```python
from build123d import *

# Parameters (mm, degrees)
BOSS_EXTRUDE6_DEPTH = 4
CUT_EXTRUDE1_DEPTH  = 2


with BuildPart() as part:
    # Sketch2 → Boss-Extrude6 (new body)
    with BuildSketch(Plane.XY):
        with BuildLine():
            Line((7.936945185, 4.607509822), (-12.657523049, 2.384648727))
            ThreePointArc((-12.657523049, 2.384648727), (-14.798635322, 0), (-12.657523049, -2.384648727))
            Line((-12.657523049, -2.384648727), (7.936945185, -4.607509822))
            ThreePointArc((7.936945185, -4.607509822), (18.479455181, 0), (7.936945185, 4.607509822))
        make_face()
    extrude(amount=BOSS_EXTRUDE6_DEPTH)

    # Sketch1 → Cut-Extrude1 (cut)
    with BuildSketch(Plane.XY):
        with BuildLine():
            Line((-2.308259951, 2.498066053), (9.375044145, 3.190055955))
            add(Edge.make_bspline(
                [(9.375044145, 3.190055955), (9.743762717, 3.535051607), (10.542113364, 3.885379294), (11.739855888, 4.053778423), (12.781606273, 3.904003548), (13.647647588, 3.58835165), (14.172524986, 3.123610305), (14.749448402, 2.727996587), (15.239395752, 2.01553181), (15.653528757, 1.050879588), (15.788992815, -0.000691818), (15.651665108, -1.048112313), (15.246850359, -2.025217286), (14.603250264, -2.863967716), (13.764299096, -3.507779486), (12.787785525, -3.91194775), (11.73820132, -4.051651269), (10.542857019, -3.886335356), (9.743600409, -3.534842939), (9.375044145, -3.190055955)],
                knots=[0, 0, 0, 0, 0.085136877, 0.144403023, 0.203669169, 0.262935434, 0.297502717, 0.322201499, 0.3814676, 0.440733879, 0.5, 0.559266121, 0.6185324, 0.677798501, 0.737064566, 0.796330831, 0.855596977, 0.914863123, 1, 1, 1, 1], degree=3))
            Line((9.375044145, -3.190055955), (-2.308259951, -2.498066053))
            add(Edge.make_bspline(
                [(-2.308259951, -2.498066053), (-2.730270965, -2.498681523), (-3.365255191, -2.317767142), (-4.051947117, -1.791219452), (-4.45450445, -1.266528616), (-4.707556493, -0.655614107), (-4.793872131, 0), (-4.707556493, 0.655614107), (-4.45450445, 1.266528616), (-4.051947117, 1.791219452), (-3.365255191, 2.317767142), (-2.730270965, 2.498681523), (-2.308259951, 2.498066053)],
                knots=[0, 0, 0, 0, 0.162547316, 0.2469105, 0.331273485, 0.415637006, 0.5, 0.584362994, 0.668726515, 0.7530895, 0.837452684, 1, 1, 1, 1], degree=3))
        make_face()
    extrude(amount=CUT_EXTRUDE1_DEPTH, mode=Mode.SUBTRACT)


solid = part.part
```
The listing builds one solid part. Answer for the finished solid, in the listing's coordinates (mm). A direction names the side the tool comes from. Round coordinates to 2 decimals unless told otherwise and drop trailing zeros. Loops run counter-clockwise (first coordinate to the right, second up) from the corner with the lowest first, then second, coordinate; pieces in that order, holes last. Notation, with made-up numbers: (-14.75, 42) -> (0.25, 42) arc R19 cw to (0.25, 65) -> close; hole circle Ø5 at (44, 38.25). An arc over 180 degrees is marked (long way). Use one line per item in the form item = value.
1. A tool of negligible diameter and unlimited length cuts with its end or side. For faces 5 (the flat face through (6, 0, 2)), 6 (the flat face through (-2.22, 3.51, 1.97)), from which of +Z, -Z, +X, -X, +Y, -Y can it reach the whole face along a straight path? Write none if from no direction.
Answer key:
face_5 = -Z
face_6 = +Z, -Z, -X, +Y
2. For a pull along X with two mould halves and no side action, classify faces 1 (the flat face through (-2.5, -3.48, 1.97)), 2 (the flat face through (3.45, 2.84, 0.99)), 3 (the flat face through (3.62, -2.85, 0.99)), 4 (the cylindrical face through (18.476, -0.204, 1.972)) as released by +X, released by -X, zero draft, split by the parting line, or undercut.
Answer key:
face_1 = released by -X
face_2 = undercut
face_3 = undercut
face_4 = split by the parting line
3. Flat-ended cylindrical pins translate along their axes: pin 1 Ø1 at (x, z) = (1.5, 1) entering from -Y; pin 2 Ø1.5 at (x, y) = (13, 0) entering from -Z. Find the tip coordinate at first contact, or state that the pin passes through.
Answer key:
pin_1 = -3.97
pin_2 = 2
4. Find the intervals of material crossed by probe 1 along X at (y, z) = (-1, 1); probe 2 along Y at (x, z) = (-1, 1.75); probe 3 along Y at (x, z) = (10.5, 1.15), in increasing order. Write a range as [from, to].
Answer key:
probe_1 = [-14.58, -4.56], [15.62, 18.4]
probe_2 = [-3.64, -2.58], [2.58, 3.64]
probe_3 = [-6.04, -3.81], [3.81, 6.04]
5. The part is cut by section C-C on y = -5.5. Determine the outline of the cut face in (x, z).
Answer key:
outline = (9.17, 0) -> (15.23, 0) -> (15.23, 4) -> (9.17, 4) -> close
6. The part is cut by section B-B on x = 3.5. Determine the outline of the cut face in (y, z), and give its area (3 significant figures).
Answer key:
outline = (-4.13, 0) -> (-2.84, 0) -> (-2.84, 2) -> (2.84, 2) -> (2.84, 0) -> (4.13, 0) -> (4.13, 4) -> (-4.13, 4) -> close
area = 21.7 mm²
7. The part is cut by section A-A on z = 2.9. Determine the outline of the cut face in (x, y).
Answer key:
outline = (-12.66, -2.38) -> (7.94, -4.61) arc R6.28 ccw (long way) to (7.94, 4.61) -> (-12.66, 2.38) arc R2.4 ccw to start
